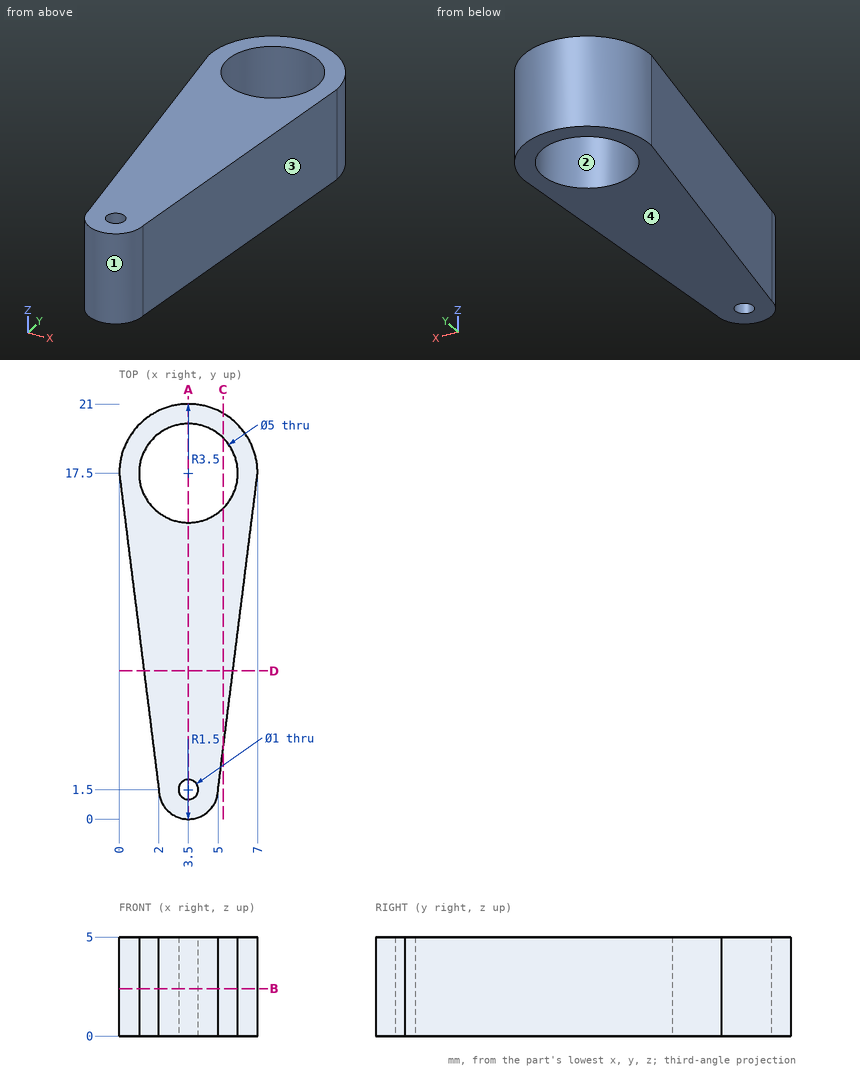
Drawing for the job (mm, zero at the part's lowest x, y, z). Give positions to 0.01 mm unless a question says otherwise; leave off trailing zeros. Write each loop counter-clockwise with the first axis right and the second up, starting at its lowest first coordinate (ties: lowest second). Pieces come first, ordered by that corner, then holes. Notation, with made-up numbers: M 62.25,76 L 114.25,76 A24 ccw 114.25,94 Z; hole C 7,19 d10. An arc over 180 degrees is marked long. Return JSON: item names as keys, results as strings. Group by question number.
(1) Band-saw the part on A-A (x = 3.5). Give the cut face in (y, z).
(2) Band-saw the part on C-C (x = 5.25). Give the cut face in (y, z), and give its area (3 significant figures).
(3) Drill centre lines: L1, parallel to Y at x = 3.5, z = 3.4; L2, parallel to Y at x = 2.5, z = 1.95; L3, parallel to Y at x = 2.75, z = 4.35. Where is each one in solid material? Low to high. Write a range as [from, to].
(4) Mould opens along X. For the marked faces 1, 2, 3 and 4 say: pulls with the +X half, pulls with the -X half, needs draft (parallel to the pull), parting line crosses it, or undercut.
(5) Band-saw the part on D-D (y = 7.5). Give the cut face in (x, z), and give its area (3 significant figures).
(6) Band-saw the part on B-B (z = 2.4). Give the cut face in (x, y), and give its area (3 significant figures).
Entries:
{
 "1": {"outline": "M 0,0 L 1,0 L 1,5 L 0,5 Z; M 2,0 L 15,0 L 15,5 L 2,5 Z; M 20,0 L 21,0 L 21,5 L 20,5 Z"},
 "2": {"outline": "M 3.5,0 L 15.71,0 L 15.71,5 L 3.5,5 Z; M 19.29,0 L 20.53,0 L 20.53,5 L 19.29,5 Z", "area": "67.3 mm^2"},
 "3": {"L1": "y = [0, 1], [2, 15], [20, 21]", "L2": "y = [0.38, 15.21], [19.79, 20.85]", "L3": "y = [0.2, 15.12], [19.88, 20.92]"},
 "4": {"face 1": "parting line crosses it", "face 2": "undercut", "face 3": "pulls with the +X half", "face 4": "needs draft"},
 "5": {"outline": "M 1.25,0 L 5.75,0 L 5.75,5 L 1.25,5 Z", "area": "22.5 mm^2"},
 "6": {"outline": "M 0,17.5 L 2,1.5 A1.5 ccw 5,1.5 L 7,17.5 A3.5 ccw Z; hole C 3.5,17.5 d5; hole C 3.5,1.5 d1", "area": "82.4 mm^2"}
}
